Design review of the part built by this model. Coordinates are the model's own, in mm. A direction names the side the tool comes from. Round coordinates to 2 decimals unless told otherwise and drop trailing zeros. Write each loop counter-clockwise with the first axis right and the second up, starting at its lowest first coordinate (ties: lowest second). Pieces come first, ordered by that corner, then holes. Notation, with made-up numbers: M 21.5,-11 L 44.5,-11 A26 cw 44.5,16 Z; hole C 22,2.25 d10. An arc over 180 degrees is marked long. Use CSV: the item, a comma, the result in double quotes.
from build123d import *

# Parameters (mm, degrees)
BOSS_EXTRUDE1_DEPTH          = 15
SKETCH4_R                    = 20
CUT_EXTRUDE1_DEPTH           = 30
SKETCH5_R                    = 40
CUT_EXTRUDE2_DEPTH           = 18
M10_TAPPED_HOLE1_D           = 8.5
M10_TAPPED_HOLE1_DEPTH       = 24.5
M10_TAPPED_HOLE1_CSINK_D     = 10.05
M10_TAPPED_HOLE1_CSINK_ANGLE = 90
M10_TAPPED_HOLE1_TIP         = 2.553657631


with BuildPart() as part:
    # Sketch2 → Boss-Extrude1 (new, symmetric)
    with BuildSketch(Plane.XY):
        with BuildLine():
            Line((-50, 0), (-50, 80))
            Line((-50, 80), (50, 80))
            Line((50, 80), (50, 0))
            ThreePointArc((50, 0), (0, -50), (-50, 0))
        make_face()
    extrude(amount=BOSS_EXTRUDE1_DEPTH, both=True)

    # Sketch4 → Cut-Extrude1 (cut)
    with BuildSketch(Plane.XY.offset(15)):
        Circle(SKETCH4_R)
    extrude(amount=-CUT_EXTRUDE1_DEPTH, mode=Mode.SUBTRACT)

    # Sketch5 → Cut-Extrude2 (cut)
    with BuildSketch(Plane.XY.offset(15)):
        Circle(SKETCH5_R)
    extrude(amount=-CUT_EXTRUDE2_DEPTH, mode=Mode.SUBTRACT)

    # M10 Tapped Hole1
    with Locations(Plane(origin=(-35, 80, 0), x_dir=(0, 0, 1), z_dir=(0, 1, 0))):
        with Locations((0, 0), (0, 70)):
            CounterSinkHole(M10_TAPPED_HOLE1_D / 2, M10_TAPPED_HOLE1_CSINK_D / 2, depth=M10_TAPPED_HOLE1_DEPTH, counter_sink_angle=M10_TAPPED_HOLE1_CSINK_ANGLE)
            with Locations((0, 0, -(M10_TAPPED_HOLE1_DEPTH + M10_TAPPED_HOLE1_TIP / 2))):  # 118° drill point
                Cone(0, M10_TAPPED_HOLE1_D / 2, M10_TAPPED_HOLE1_TIP, mode=Mode.SUBTRACT)


solid = part.part
1) Add section D-D on y = -31. Write out the cut boundary in (x, z).
Answers:
outline,"M -39.23,-15 L 39.23,-15 L 39.23,15 L 25.28,15 L 25.28,-3 L -25.28,-3 L -25.28,15 L -39.23,15 Z"
2) For pin 1 Ø10 at (x, z) = (-35, 0) entering from +Y (3 decimals); pin 2 Ø12 at (x, z) = (23.5, -1.5) entering from -Y; pin 3 Ø5 at (x, z) = (-30.5, -10.5) entering from -Y, all flat-tipped, find the tip position at first contact; note any pin that passes through.
Answers:
pin 1,"y = 79.975"
pin 2,"y = -46.84"
pin 3,"y = -41.42"
3) Add section A-A on x = 0. Write out the cut boundary in (y, z), then the cut area to 3 significant figures.
Answers:
outline,"M -50,-15 L -20,-15 L -20,-3 L -40,-3 L -40,15 L -50,15 Z; M 20,-15 L 80,-15 L 80,15 L 40,15 L 40,-3 L 20,-3 Z"
area,"1,980 mm²"
4) Wall thickness on line 1 along X through (y, z) = (69.5, 0); line 2 along Y through (x, z) = (0, -7.25); line 3 along Y through (x, z) = (0, 8): over which ranges is each line inside the solid? List them lowest first. Write a range as [from, to].
Answers:
line 1,"[-50, -39.25], [-30.75, 30.75], [39.25, 50]"
line 2,"[-50, -20], [20, 80]"
line 3,"[-50, -40], [40, 80]"
5) The part is to be moulded in two halves that separate along Y. For faces 4 (the face through (-4.336, -19.524, -8.916)), 5 (the face through (1, 30, -15)), 6 (the face through (34.345, 53.39, 0.341)), say which applies: released by +Y, released by -Y, zero draft, split by the parting line, or undercut.
Answers:
face 4,"undercut"
face 5,"zero draft"
face 6,"released by +Y"
6) Add section C-C on y = 9. Write out the cut boundary in (x, z).
Answers:
outline,"M -50,-15 L -17.86,-15 L -17.86,-3 L -38.97,-3 L -38.97,15 L -50,15 Z; M 17.86,-15 L 50,-15 L 50,15 L 38.97,15 L 38.97,-3 L 17.86,-3 Z"
7) Add section B-B on z = -6.5. Write out the cut boundary in (x, y).
Answers:
outline,"M -50,0 A50 ccw 50,0 L 50,80 L -50,80 Z; hole C 0,0 d40"
8) Machinability: for faces 1 (the face through (39.214, 67.196, 0.553)), 2 (the face through (-8.67, -39.05, 6.13)), 3 (the face through (50, 41, 0)), which of the approach directions +Z, -Z, +X, -X, +Y, -Y give a long, thin tool a straight path to every point of the face, cutting with its end or side? Answer none if there is none.
Answers:
face 1,"+Y"
face 2,"+Z"
face 3,"+Z, -Z, +X, +Y, -Y"
